```python
from build123d import *

# Parameters (mm, degrees)
SKETCH_1_W          = 105
SKETCH_1_H          = 24
EXTRUDE_1_DEPTH     = 35
SKETCH_2_W          = 33
SKETCH_2_H          = 20.5
CUT_EXTRUDE_1_DEPTH = 50
CUT_EXTRUDE_2_DEPTH = 55


with BuildPart() as part:
    # 草图1 → 凸台-拉伸1 (new body)
    with BuildSketch(Plane.XY):
        with Locations((-16.041666667, 6.034090909)):
            Rectangle(SKETCH_1_W, SKETCH_1_H)
    extrude(amount=EXTRUDE_1_DEPTH)

    # 草图2 → 切除-拉伸1 (cut)
    with BuildSketch(Plane.ZY.offset(68.541666667)):
        with Locations((16.5, 6.034090909)):
            Rectangle(SKETCH_2_W, SKETCH_2_H)
    extrude(amount=-CUT_EXTRUDE_1_DEPTH, mode=Mode.SUBTRACT)

    # 草图3 → 切除-拉伸2 (cut)
    with BuildSketch(Plane(origin=(36.458333333, 0, 0), x_dir=(0, 0, -1), z_dir=(1, 0, 0))):
        Polygon((-33, 16.284090909), (-4, 16.284090909), (-4, 18.034090909), (0, 18.034090909), (0, -5.965909091), (-4, -5.965909091), (-4, -4.215909091), (-33, -4.215909091), align=None)
    extrude(amount=-CUT_EXTRUDE_2_DEPTH, mode=Mode.SUBTRACT)


solid = part.part
```
Source: CAD feature listing. Evaluate the final solid. Frame: model axes, mm. A direction names the side the tool comes from. Round coordinates to 2 decimals unless told otherwise and drop trailing zeros. Write each loop counter-clockwise with the first axis right and the second up, starting at its lowest first coordinate (ties: lowest second). Pieces come first, ordered by that corner, then holes. Notation, with made-up numbers: M -29,-23 L -21,-23 A27 ccw -21,15 Z; hole C 55,72 d3. An arc over 180 degrees is marked long. Answer as a JSON object with one key per item and string values. Group by question number.
(1) First-contact query: pin 1 (2 mm diameter, centred on x = 26, y = 12, fed in from -Z); pin 2 (1.4 mm diameter, centred on y = 17.5, z = 2.5, fed in from +X); pin 3 (1.4 mm diameter, centred on x = 0, y = 17, fed in from -Z). Flat tips, straight axial feed; report the tip coordinate or a pass-through.
(2) Reachability of faces 1 (the flat face through (9, 17, 4)), 2 (the flat face through (-68.542, -5, 21)), 3 (the flat face through (-17, 6, 33)) from +Z, -Z, +X, -X, +Y, -Y: full face, straight path, thin tool, end or side. Return the list, or none.
(3) Ray query, line 1 (Y direction, x = 25.5, z = 29); line 2 (Z direction, x = -53, y = 0.25); line 3 (Z direction, x = 3, y = -4.75). Return the intervals inside material, ascending. Write a range as [from, to].
(4) Section query D-D on x = 3.5. Output: boundary loops of the cut face in (y, z).
(5) Section query C-C on y = 0. Output: boundary loops of the cut face in (x, z), then the cut area to 3 significant figures.
(6) Section query B-B on x = -60. Output: boundary loops of the cut face in (y, z), then the cut area to 4 significant figures.
(7) Mould query, pull axis Y, two halves, no side actions, for faces 4 (the flat face through (-17, -4.216, 16)), 5 (the flat face through (-17, 18.034, 17)), 6 (the flat face through (-18.542, 17, 2)), 7 (the flat face through (-17, 16.284, 16)). Classes: +Y half, -Y half, draft (parallel to the pull), parting line (faces both ways), or undercut.
(8) Section query A-A on z = 23.5. Output: boundary loops of the cut face in (x, y).
Computed values:
{
 "1": {"pin 1": "z = 33", "pin 2": "x = -18.54", "pin 3": "z = 4"},
 "2": {"face 1": "-Z, +X, +Y, -Y", "face 2": "+Z, -Z, -X, +Y, -Y", "face 3": "-Z, +X, -X"},
 "3": {"line 1": "[-5.97, -4.22], [16.28, 18.03]", "line 2": "[33, 35]", "line 3": "[4, 35]"},
 "4": {"outline": "M -5.97,4 L -4.22,4 L -4.22,33 L 16.28,33 L 16.28,4 L 18.03,4 L 18.03,35 L -5.97,35 Z"},
 "5": {"outline": "M -68.54,33 L 36.46,33 L 36.46,35 L -68.54,35 Z", "area": "210 mm^2"},
 "6": {"outline": "M -5.97,0 L -4.22,0 L -4.22,33 L 16.28,33 L 16.28,0 L 18.03,0 L 18.03,35 L -5.97,35 Z", "area": "163.5 mm^2"},
 "7": {"face 4": "undercut", "face 5": "+Y half", "face 6": "draft", "face 7": "undercut"},
 "8": {"outline": "M -68.54,-5.97 L 36.46,-5.97 L 36.46,-4.22 L -68.54,-4.22 Z; M -68.54,16.28 L 36.46,16.28 L 36.46,18.03 L -68.54,18.03 Z"}
}
